from build123d import *

# Parameters (mm, degrees)
F0_W     = 311.15
F0_H     = 121.4
F0_R     = 2.5
F0_R_2   = 2
F1_DEPTH = 13
F2_T     = -1
F4_DEPTH = 17
F5_DEPTH = 17
F6_DEPTH = 17
F7_DEPTH = 17


# Not quite as in the source:
# - the program builds the solid bodies; features that only make, move or delete a surface that nothing else refers to are left out


with BuildPart() as f1:
    # F0 (on Top) → F1 (new body)
    with BuildSketch(Plane.XY):
        with Locations((6.6334828734, -24.2652736852)):
            Rectangle(F0_W, F0_H)
        with Locations((-116.9415171266, -32.9652736852)):
            Circle(F0_R, mode=Mode.SUBTRACT)
        with Locations((-61.4415171266, -23.5952736852)):
            Circle(F0_R_2, mode=Mode.SUBTRACT)
        with Locations((74.7084828734, -23.5652736852)):
            Circle(F0_R_2, mode=Mode.SUBTRACT)
        with Locations((114.5584828734, -13.7852736852)):
            Circle(F0_R, mode=Mode.SUBTRACT)
        with Locations((-116.9415171266, -32.9652736852)):
            Circle(F0_R)
        with Locations((114.5584828734, -13.7852736852)):
            Circle(F0_R)
        with Locations((-61.4415171266, -23.5952736852)):
            Circle(F0_R_2)
        with Locations((74.7084828734, -23.5652736852)):
            Circle(F0_R_2)
    extrude(amount=F1_DEPTH)

    # F2
    f2_openings = [f1.faces().sort_by_distance(p)[0] for p in [
        (6.633483, -24.265274, 13),
    ]]
    offset(amount=F2_T, openings=f2_openings)

    # F4 (add): a face of the model
    f4_faces = [f1.faces().sort_by_distance(p)[0] for p in [
        (6.6334828734, -84.9652736852, 6.5),
    ]]
    extrude(f4_faces, amount=F4_DEPTH)

    # F5 (add): a face of the model
    f5_faces = [f1.faces().sort_by_distance(p)[0] for p in [
        (-148.9415171266, -32.7652736852, 6.5),
    ]]
    extrude(f5_faces, amount=F5_DEPTH)

    # F6 (add): a face of the model
    f6_faces = [f1.faces().sort_by_distance(p)[0] for p in [
        (162.2084828734, -32.7652736852, 6.5),
    ]]
    extrude(f6_faces, amount=F6_DEPTH)

    # F7 (add): a face of the model
    f7_faces = [f1.faces().sort_by_distance(p)[0] for p in [
        (6.6334828734, 36.4347263148, 6.5),
    ]]
    extrude(f7_faces, amount=F7_DEPTH)


solid = f1.part
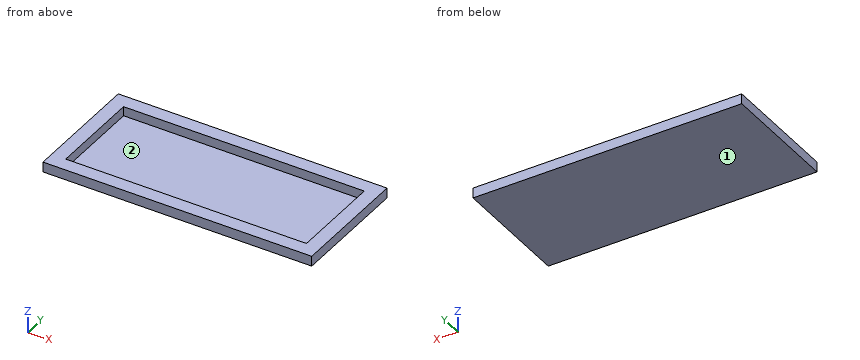
Here's how the part is built. I have some questions about the finished solid (model axes, mm). Face numbers are marked on the shaded views. Round coordinates to 2 decimals unless told otherwise and drop trailing zeros. Write each loop counter-clockwise with the first axis right and the second up, starting at its lowest first coordinate (ties: lowest second). Pieces come first, ordered by that corner, then holes.
1. I need wall thicknesses on L1, parallel to Y at x = 116, z = 4.75; L2, parallel to X at y = -21, z = 9; L3, parallel to Z at x = -117.5, y = -8. Which ranges of each line are inside material? Lowest first, please.
2. Will this pin go through, and if not, where does the flat tip stop? pin 1 Ø1.5 at (x, y) = (27, 5.5) entering from -Z.
3. Suppose I cut it at B-B (y = 8.5). List the corners of the cut face in (x, z) for me, and give its area (3 significant figures).
4. If we mould it in two halves opening along Y, with no side actions, what happens to the marked faces 1 and 2? For each: released by +Y, released by -Y, zero draft, split by the parting line, or undercut.
5. Suppose I cut it at C-C (z = 5.25). List the corners of the cut face in (x, y) for me.
6. Suppose I cut it at A-A (x = -58.5). List the corners of the cut face in (y, z) for me, and give its area (3 significant figures).
Answer sheet:
1. L1: y = -101.97 to -83.97, 35.43 to 53.43
1. L2: x = -165.94 to -147.94, 161.21 to 179.21
1. L3: z = 0 to 1
2. pin 1: stops at z = 0
3. outline: (-165.94, 0) - (179.21, 0) - (179.21, 13) - (161.21, 13) - (161.21, 1) - (-147.94, 1) - (-147.94, 13) - (-165.94, 13) - close
3. area: 777 mm2
4. face 1: zero draft
4. face 2: undercut
5. outline: (-165.94, -101.97) - (179.21, -101.97) - (179.21, 53.43) - (-165.94, 53.43) - close; hole (-147.94, -83.97) - (161.21, -83.97) - (161.21, 35.43) - (-147.94, 35.43) - close
6. outline: (-101.97, 0) - (53.43, 0) - (53.43, 13) - (35.43, 13) - (35.43, 1) - (-83.97, 1) - (-83.97, 13) - (-101.97, 13) - close
6. area: 587 mm2
